from build123d import *

# Parameters (mm, degrees)
F2_R     = 10
F3_DEPTH = 26
F4_R     = 2.5
F4_R_2   = 10
F5_DEPTH = 15
F6_R     = 5
F7_R     = 0.5
F8_R     = 4
F9_DEPTH = 2


with BuildPart() as f1:
    # F0 (on Top) → F1 (revolve)
    with BuildSketch(Plane.XY):
        with BuildLine():
            ThreePointArc((-12.5, 0), (0, -12.5), (12.5, 0))
            Line((12.5, 0), (-12.5, 0))
        make_face()
    revolve(axis=Axis((5, 0, 0), (-1, 0, 0)))

    # F2 (on Top) → F3 (join)
    with BuildSketch(Plane.XY):
        Circle(F2_R)
    extrude(amount=-F3_DEPTH)

    # F4 (on face) → F5 (join)
    with BuildSketch(Plane(origin=(0, 0, -26), x_dir=(1, 0, 0), z_dir=(0, 0, -1))):
        Polygon((7, 15), (0, 15), (-7, 15), (-22, 0), (-7, -15), (0, -15), (7, -15), (22, 0), align=None)
        with Locations((-15, 0)):
            Circle(F4_R, mode=Mode.SUBTRACT)
        Circle(F4_R_2, mode=Mode.SUBTRACT)
        with Locations((15, 0)):
            Circle(F4_R, mode=Mode.SUBTRACT)
    extrude(amount=-F5_DEPTH)

    # F6
    f6_edges = [f1.edges().sort_by_distance(p)[0] for p in [
        (-22, 0, -18.5),
        (-7, -15, -18.5),
        (7, -15, -18.5),
        (22, 0, -18.5),
        (7, 15, -18.5),
        (-7, 15, -18.5),
    ]]
    fillet(f6_edges, radius=F6_R)

    # F7
    f7_edges = [f1.edges().sort_by_distance(p)[0] for p in [
        (-13.464466, -8.535534, -11),
    ]]
    fillet(f7_edges, radius=F7_R)

    # F8 (on face) → F9 (cut)
    with BuildSketch(Plane.XY.offset(-11)):
        with Locations((-14.928932, 0)):
            Circle(F8_R)
        with Locations((15, 0)):
            Circle(F8_R)
    extrude(amount=-F9_DEPTH, mode=Mode.SUBTRACT)


solid = f1.part
The model under review builds one solid part; all positions refer to its coordinate system, in mm. A direction names the side the tool comes from. Coordinates: 2 decimals unless noted, no trailing zeros. Write each loop counter-clockwise with the first axis right and the second up, starting at its lowest first coordinate (ties: lowest second). Pieces come first, ordered by that corner, then holes. Notation, with made-up numbers: (-14.5, 78) -> (19.5, 78) arc R31 ccw to (19.5, 107) -> close; hole circle Ø6 at (87, -18.75). An arc over 180 degrees is marked (long way). Answer in a Markdown table with one row per item.
1. We need section D-D, the plane z = 10.5. State the section outline as (x, y) points, and give its area (3 significant figures).
Answers below:
| item | result |
|---|---|
| outline | circle Ø13.56 at (0, 0) |
| area | 145 mm^2 |
2. We need section B-B, the plane x = 0. State the section outline as (y, z) points.
Answers below:
| item | result |
|---|---|
| outline | (-15, -26) -> (15, -26) -> (15, -11.5) arc R0.5 ccw to (14.5, -11) -> (10, -11) -> (10, -7.5) arc R12.5 ccw (long way) to (-10, -7.5) -> (-10, -11) -> (-14.5, -11) arc R0.5 ccw to (-15, -11.5) -> close |
3. Wall thickness on probe 1 along X at (y, z) = (0, -19.5); probe 2 along X at (y, z) = (2, -15); probe 3 along Z at (x, y) = (10, -8): over which ranges is each line inside the solid? List them lowest first. Write a range as [from, to].
Answers below:
| item | result |
|---|---|
| probe 1 | x = [-19.93, -17.5], [-12.5, 12.5], [17.5, 19.93] |
| probe 2 | x = [-19.51, -16.5], [-13.5, 13.5], [16.5, 19.51] |
| probe 3 | z = [-26, -11] |
4. Draft analysis for pull direction Y (two halves, no side actions). For faces 3 (the cylindrical face through (-17.5, -0.1, -19.6)), 4 (the flat face through (-10.2, -0.1, -11)), 5 (the flat face through (-14, 8, -19)), 6 (the cylindrical face through (6.82, -14.63, -18.65)), state which applies: +Y half, -Y half, draft (parallel to the pull), parting line (faces both ways), or undercut.
Answers below:
| item | result |
|---|---|
| face 3 | undercut |
| face 4 | draft |
| face 5 | +Y half |
| face 6 | -Y half |
5. Clearance check with flat-ended pins moving along their axes: pin 1 Ø1.5 at (x, z) = (-12.5, -5.5) entering from -Y; pin 2 Ø6 at (y, z) = (4.5, -13.5) entering from +X; pin 3 Ø4 at (x, z) = (0, -1) entering from +Y; pin 4 Ø2.5 at (x, y) = (-14, 1) entering from +Z. State where each tip first meets the part, or that it passes through.
Answers below:
| item | result |
|---|---|
| pin 1 | passes through |
| pin 2 | stops at x = 19.7 |
| pin 3 | stops at y = 12.5 |
| pin 4 | stops at z = -13 |
6. We need section C-C, the plane z = -9. State the section outline as (x, y) points, and give its area (3 significant figures).
Answers below:
| item | result |
|---|---|
| outline | circle Ø20 at (0, 0) |
| area | 314 mm^2 |
7. For faces 1 (the cylindrical face through (-19.93, -0.05, -18.65)), 2 (the cylindrical face through (11, 0, -12)), list the 3-axis set-ups (+Z, -Z, +X, -X, +Y, -Y) from which the entire face can be reached by the end or side of a thin tool; tool diameter is ignored.
Answers below:
| item | result |
|---|---|
| face 1 | +Z, -Z, -X |
| face 2 | none |
8. We need section A-A, the plane z = -22. State the section outline as (x, y) points.
Answers below:
| item | result |
|---|---|
| outline | (-18.46, -3.54) -> (-8.46, -13.54) arc R5 ccw to (-4.93, -15) -> (4.93, -15) arc R5 ccw to (8.46, -13.54) -> (18.46, -3.54) arc R5 ccw to (18.46, 3.54) -> (8.46, 13.54) arc R5 ccw to (4.93, 15) -> (-4.93, 15) arc R5 ccw to (-8.46, 13.54) -> (-18.46, 3.54) arc R5 ccw to start; hole circle Ø5 at (-15, 0); hole circle Ø5 at (15, 0) |
